Can you work these out from the model? Positions are in its coordinate system, mm. A direction names the side the tool comes from. Give positions to 0.01 mm unless a question says otherwise; leave off trailing zeros. Loops run counter-clockwise (first coordinate to the right, second up) from the corner with the lowest first, then second, coordinate; pieces in that order, holes last. Notation, with made-up numbers: (78, 75.5) - (105, 75.5) arc R6 ccw to (105, 79.5) - close; hole circle Ø9 at (-19, 0). An arc over 180 degrees is marked (long way). Use a Markdown table: item, result. Add a question column.
```python
from build123d import *

# Parameters (mm, degrees)
SKETCH_1_R      = 4
EXTRUDE_1_DEPTH = 4


with BuildPart() as part:
    # 草图1 → 凸台-拉伸1 (new body)
    with BuildSketch(Plane.XY):
        with BuildLine():
            ThreePointArc((34.064306358, 2.179556892), (9.237186096, 7.048826392), (-4.8, -14))
            Line((-4.8, -14), (-4.8, -18.23))
            Line((-4.8, -18.23), (-7.8, -18.23))
            Line((-7.8, -18.23), (-7.8, -23.23))
            Line((-7.8, -23.23), (-4.8, -23.23))
            Line((-4.8, -23.23), (-4.8, -27.46))
            Line((-4.8, -27.46), (-7.8, -27.46))
            Line((-7.8, -27.46), (-7.8, -32.46))
            Line((-7.8, -32.46), (-4.8, -32.46))
            Line((-4.8, -32.46), (-4.8, -36.69))
            Line((-4.8, -36.69), (-7.8, -36.69))
            Line((-7.8, -36.69), (-7.8, -41.69))
            Line((-7.8, -41.69), (-4.8, -41.69))
            Line((-4.8, -41.69), (-4.8, -46.02))
            Line((-4.8, -46.02), (4.8, -46.02))
            Line((4.8, -46.02), (4.8, -41.49))
            Line((4.8, -41.49), (7.8, -41.49))
            Line((7.8, -41.49), (7.8, -36.49))
            Line((7.8, -36.49), (4.8, -36.49))
            Line((4.8, -36.49), (4.8, -32.26))
            Line((4.8, -32.26), (7.8, -32.26))
            Line((7.8, -32.26), (7.8, -27.26))
            Line((7.8, -27.26), (4.8, -27.26))
            Line((4.8, -27.26), (4.8, -23.03))
            Line((4.8, -23.03), (7.8, -23.03))
            Line((7.8, -23.03), (7.8, -18.23))
            Line((7.8, -18.23), (4.8, -18.23))
            Line((4.8, -18.23), (4.8, -13.8))
            ThreePointArc((4.8, -13.8), (6.264466094, -10.264466094), (9.8, -8.8))
            Line((9.8, -8.8), (18, -8.8))
            Line((18, -8.8), (29.480940848, -8.8))
            ThreePointArc((29.480940848, -8.8), (35.465961002, -4.851988259), (34.064306358, 2.179556892))
        make_face()
        with Locations((18, 0)):
            Circle(SKETCH_1_R, mode=Mode.SUBTRACT)
    extrude(amount=EXTRUDE_1_DEPTH)


solid = part.part
```
1. Suppose I cut it at A-A (x = 18). List the corners of the cut face in (y, z) for me, and give its area (3 significant figures).
2. Suppose I cut it at D-D (x = 6.5). List the corners of the cut face in (y, z) for me, and give its area (3 significant figures).
3. Suppose I cut it at B-B (y = -3). List the corners of the cut face in (x, z) for me, and give its area (3 significant figures).
4. If we mould it in two halves opening along X, with no side actions, what happens to faces 1 (the face through (6, -36.49, 2)), 2 (the face through (4.8, -16, 2)), 3 (the face through (14, 0, 2))? For each: released by +X, released by -X, zero draft, split by the parting line, or undercut.
5. On a 3-axis mill with a long thin cutter (end or side, diameter ignored), from which of +Z, -Z, +X, -X, +Y, -Y can I reach the whole of each face in a straight line? I mean faces 4 (the face through (-6, -41.69, 2)), 5 (the face through (6, -23.03, 2)), 6 (the face through (-6, -36.69, 2)). Say none if no direction works.
6. Will these pins go through, and if not, where does the flat tip stop? P1, Ø1.2, axis at y = -30, z = 2, coming from the +X side; P2, Ø1.5, axis at x = -6, z = 2.5, coming from the -Y side; P3, Ø0.9, axis at x = 6.5, z = 2.5, coming from the -Y side.
7. Please list where these lines run through material, in increasing order: line 1 along Y through (x, z) = (18, 2.6); line 2 along Y through (x, z) = (7.5, 2.9); line 3 along X through (y, z) = (-3, 2.1). Write a range as [from, to].
Results below:
| question | item | result |
|---|---|---|
| 1 | outline | (-8.8, 0) - (-4, 0) - (-4, 4) - (-8.8, 4) - close; (4, 0) - (8.8, 0) - (8.8, 4) - (4, 4) - close |
| 1 | area | 38.4 mm² |
| 2 | outline | (-41.49, 0) - (-36.49, 0) - (-36.49, 4) - (-41.49, 4) - close; (-32.26, 0) - (-27.26, 0) - (-27.26, 4) - (-32.26, 4) - close; (-23.03, 0) - (-18.23, 0) - (-18.23, 4) - (-23.03, 4) - close; (-10.04, 0) - (5.69, 0) - (5.69, 4) - (-10.04, 4) - close |
| 2 | area | 122 mm² |
| 3 | outline | (-1.97, 0) - (15.35, 0) - (15.35, 4) - (-1.97, 4) - close; (20.65, 0) - (35.93, 0) - (35.93, 4) - (20.65, 4) - close |
| 3 | area | 130 mm² |
| 4 | face 1 | zero draft |
| 4 | face 2 | released by +X |
| 4 | face 3 | undercut |
| 5 | face 4 | +Z, -Z, -X, -Y |
| 5 | face 5 | +Z, -Z, +X |
| 5 | face 6 | +Z, -Z, -X |
| 6 | P1 | x = 7.8 |
| 6 | P2 | y = -41.69 |
| 6 | P3 | y = -41.49 |
| 7 | line 1 | [-8.8, -4], [4, 8.8] |
| 7 | line 2 | [-41.49, -36.49], [-32.26, -27.26], [-23.03, -18.23], [-9.36, 6.24] |
| 7 | line 3 | [-1.97, 15.35], [20.65, 35.93] |
